from build123d import *

# Parameters (mm, degrees)
F0_W     = 600
F0_H     = 300
F0_R     = 120
F1_DEPTH = 10
F0_R_2   = 110
F2_DEPTH = 5
F3_W     = 600
F3_H     = 10
F4_DEPTH = 10


# Not quite as in the source:
# - a feature names something its author has since deleted; it is built from what else it names


with BuildPart() as f1:
    # F0 (on Top) → F1 (new body)
    with BuildSketch(Plane.XY):
        Rectangle(F0_W, F0_H)
        Circle(F0_R, mode=Mode.SUBTRACT)
    extrude(amount=F1_DEPTH)

    # F0 (on Top) → F2 (join)
    with BuildSketch(Plane.XY):
        Circle(F0_R)
        Circle(F0_R_2, mode=Mode.SUBTRACT)
    extrude(amount=F2_DEPTH)

    # F3 (on face) → F4 (join)
    with BuildSketch(Plane.XY):
        with Locations((0, -145)):
            Rectangle(F3_W, F3_H)
        with Locations((0, -155)):
            Rectangle(F3_W, F3_H)
        Polygon((300, 140), (-300, 140), (-300, 120), (-9.09e-08, 120), (300, 120), align=None)
    extrude(amount=-F4_DEPTH)


solid = f1.part
Could you check a few things on this model? Use its own coordinates, in mm. A direction names the side the tool comes from. Coordinates: 2 decimals unless noted, no trailing zeros. Loops run counter-clockwise (first coordinate to the right, second up) from the corner with the lowest first, then second, coordinate; pieces in that order, holes last.
1. We'd pull the mould along Y, two halves only. Please class faces 1 (the face through (-4, 130, -10)), 2 (the face through (53, -97, 5)): released by +Y, released by -Y, zero draft, split by the parting line, or undercut.
2. Imagine slicing it at D-D (y = -103). Please give me the cut outline in (x, z).
3. Imagine slicing it at B-B (x = 0). Please give me the cut outline in (y, z), and give its area (3 significant figures).
4. Imagine slicing it at A-A (y = 0). Please give me the cut outline in (x, z).
5. For faces 3 (the face through (-119.884, 5.276, 7.465)), 4 (the face through (-71, -95, 0)), 5 (the face through (300, -7, 2)), which set-ups out of +Z, -Z, +X, -X, +Y, -Y let a thin tool reach every point of the face, with its end or its side?
6. I need wall thicknesses on L1, parallel to Y at x = -24, z = -1.75; L2, parallel to Y at x = 0, z = 7.2; L3, parallel to Y at x = -170, z = 3. Which ranges of each line are inside material? Lowest first, please.
7. Imagine slicing it at C-C (x = 228.5). Please give me the cut outline in (y, z), and give its area (3 significant figures).
8. For P1, Ø5, axis at x = -101.5, y = -154, coming from the +Z side; P2, Ø4, axis at x = 229, y = -124, coming from the -Z side; P3, Ø5, axis at x = -86, z = 5.5, coming from the -Y side, each with a flat end and sliding along its axis, tell me the tip position at first contact or that it passes through.
Computed values:
1. face 1: zero draft
1. face 2: undercut
2. outline: (-300, 0) - (-38.61, 0) - (-38.61, 5) - (-61.57, 5) - (-61.57, 10) - (-300, 10) - close; (38.61, 0) - (300, 0) - (300, 10) - (61.57, 10) - (61.57, 5) - (38.61, 5) - close
3. outline: (-160, -10) - (-140, -10) - (-140, 0) - (-110, 0) - (-110, 5) - (-120, 5) - (-120, 10) - (-150, 10) - (-150, 0) - (-160, 0) - close; (110, 0) - (120, 0) - (120, -10) - (140, -10) - (140, 0) - (150, 0) - (150, 10) - (120, 10) - (120, 5) - (110, 5) - close
3. area: 1,100 mm2
4. outline: (-300, 0) - (-110, 0) - (-110, 5) - (-120, 5) - (-120, 10) - (-300, 10) - close; (110, 0) - (300, 0) - (300, 10) - (120, 10) - (120, 5) - (110, 5) - close
5. face 3: +Z
5. face 4: -Z, +X, -X
5. face 5: +Z, -Z, +X, +Y, -Y
6. L1: y = -160 to -140, 120 to 140
6. L2: y = -150 to -120, 120 to 150
6. L3: y = -150 to 150
7. outline: (-160, -10) - (-140, -10) - (-140, 0) - (120, 0) - (120, -10) - (140, -10) - (140, 0) - (150, 0) - (150, 10) - (-150, 10) - (-150, 0) - (-160, 0) - close
7. area: 3,400 mm2
8. P1: stops at z = 0
8. P2: stops at z = 0
8. P3: stops at y = -150
